```python
from build123d import *

# Parameters (mm, degrees)
EXTRUDE_1_DEPTH         = 5
SKETCH_2_R              = 14
SKETCH_2_R_2            = 12.3
EXTRUDE_2_DEPTH         = 4.5
SKETCH_3_W              = 18
SKETCH_3_H              = 18
EXTRUDE_3_DEPTH         = 3
SKETCH_4_R              = 3.6
CUT_EXTRUDE_2_DEPTH     = 24.286262044
HOLE_WIZARD_M2_1_D      = 2.4
HOLE_WIZARD_M2_1_DEPTH  = 3
HOLE_WIZARD_M2_1_TIP    = 0.721032743
CUT_EXTRUDE1_DEPTH      = 24.286262044
CUT_EXTRUDE1_DEPTH_BACK = 24.286262044
SKETCH1_R               = 1


with BuildPart() as part:
    # 스케치1 → 보스-돌출1 (new body)
    with BuildSketch(Plane.XY):
        with BuildLine():
            Line((-6, 16), (6, 16))
            ThreePointArc((6, 16), (11.656854249, 13.656854249), (14, 8))
            Line((14, 8), (14, -8))
            ThreePointArc((14, -8), (11.656854249, -13.656854249), (6, -16))
            Line((6, -16), (-6, -16))
            ThreePointArc((-6, -16), (-11.656854249, -13.656854249), (-14, -8))
            Line((-14, -8), (-14, 8))
            ThreePointArc((-14, 8), (-11.656854249, 13.656854249), (-6, 16))
        make_face()
    extrude(amount=EXTRUDE_1_DEPTH)

    # 스케치2 → 보스-돌출2 (add)
    with BuildSketch(Plane.XY.offset(5)):
        Circle(SKETCH_2_R)
        Circle(SKETCH_2_R_2, mode=Mode.SUBTRACT)
    extrude(amount=EXTRUDE_2_DEPTH)

    # 스케치3 → 보스-돌출3 (add)
    with BuildSketch(Plane(origin=(0, 0, 0), x_dir=(-1, 0, 0), z_dir=(0, 0, -1))):
        with BuildLine():
            Line((-10, 10), (-7.3, 10))
            Line((-7.3, 10), (-7.3, 14.8))
            Line((-7.3, 14.8), (-6, 14.8))
            Line((-6, 14.8), (-6, 16))
            Line((-6, 16), (6, 16))
            Line((6, 16), (6, 14.8))
            Line((6, 14.8), (7.3, 14.8))
            Line((7.3, 14.8), (7.3, 10))
            Line((7.3, 10), (10, 10))
            Line((10, 10), (10, 2.4))
            Line((10, 2.4), (11, 2.4))
            ThreePointArc((11, 2.4), (13.4, 0), (11, -2.4))
            Line((11, -2.4), (10, -2.4))
            Line((10, -2.4), (10, -10))
            Line((10, -10), (-10, -10))
            Line((-10, -10), (-10, -2.4))
            Line((-10, -2.4), (-11, -2.4))
            ThreePointArc((-11, -2.4), (-13.4, 0), (-11, 2.4))
            Line((-11, 2.4), (-10, 2.4))
            Line((-10, 2.4), (-10, 10))
        make_face()
        Rectangle(SKETCH_3_W, SKETCH_3_H, mode=Mode.SUBTRACT)
    extrude(amount=EXTRUDE_3_DEPTH)

    # 스케치4 → 컷-돌출2 (cut, through all)
    with BuildSketch(Plane.XY):
        Circle(SKETCH_4_R)
    extrude(amount=CUT_EXTRUDE_2_DEPTH, mode=Mode.SUBTRACT)

    # M2 여유 구멍1
    with Locations(Plane(origin=(-11, 0, -3), x_dir=(-1, 0, 0), z_dir=(0, 0, -1))):
        with Locations((0, 0), (-22, 0)):
            Hole(HOLE_WIZARD_M2_1_D / 2, depth=HOLE_WIZARD_M2_1_DEPTH)
            with Locations((0, 0, -(HOLE_WIZARD_M2_1_DEPTH + HOLE_WIZARD_M2_1_TIP / 2))):  # 118° drill point
                Cone(0, HOLE_WIZARD_M2_1_D / 2, HOLE_WIZARD_M2_1_TIP, mode=Mode.SUBTRACT)

    # Sketch1 → Cut-Extrude1 (cut, two sides: drawn at the far end of the back side and taken through both)
    with BuildSketch(Plane(origin=(0, 0, 0), x_dir=(1, 0, 0), z_dir=(0, 1, 0)).offset(-CUT_EXTRUDE1_DEPTH_BACK)):
        with Locations(Location((0, -7.75, 0), (0, 0, 270))):
            Circle(SKETCH1_R)
    extrude(amount=CUT_EXTRUDE1_DEPTH + CUT_EXTRUDE1_DEPTH_BACK, mode=Mode.SUBTRACT)


solid = part.part
```
Can you work these out from the model? Positions are in its coordinate system, mm. A direction names the side the tool comes from. Give positions to 0.01 mm unless a question says otherwise; leave off trailing zeros. Loops run counter-clockwise (first coordinate to the right, second up) from the corner with the lowest first, then second, coordinate; pieces in that order, holes last. Notation, with made-up numbers: M 23,80 L 33,80 A18 ccw 33,99 Z; hole C -31.5,-5 d3. An arc over 180 degrees is marked long. One line per question, with ' | ' between items. Start each with the question number.
Q1. If we section it at B-B (x = 0): State how many separate pieces and enclosed holes the cut face has, plus the area to 4 significant figures.
Q2. If we section it at A-A (z = 2.5): Please give me the cut outline in (x, y).
Q3. If we mould it in two halves opening along X, with no side actions, what happens to faces 1 (the flat face through (0, 15, 5)), 2 (the cylindrical face through (-11.594, -13.719, 2.465)), 3 (the flat face through (0, 9, -1))? For each: +X half, -X half, draft (parallel to the pull), parting line (faces both ways), or undercut.
Q4. For faces 4 (the cylindrical face through (13.4, -0.05, -1.48)), 5 (the flat face through (-6, 15, -1)), 6 (the flat face through (-10.5, -2.4, -1.5)), which set-ups out of +Z, -Z, +X, -X, +Y, -Y let a thin tool reach every point of the face, with its end or its side?
Q5. For pin 1 Ø4 at (x, y) = (-11, 0) entering from +Z; pin 2 Ø0.6 at (y, z) = (15.5, -1.5) entering from +X; pin 3 Ø1 at (x, z) = (0.5, 6.5) entering from +Y; pin 4 Ø1 at (x, z) = (-7, 5) entering from +Y, each with a flat end and sliding along its axis, tell me the tip position at first contact or that it passes through.
Q6. If I drill on line 1 (X direction, y = 0, z = -1.2); line 2 (Y direction, x = 0, z = 6); line 3 (X direction, y = 0, z = 1.95), over which ranges is the centre line in solid material (lowest first)? Write a range as from..to.
Q7. If we section it at D-D (y = 13): Please give me the cut outline in (x, z) (3 decimals).
Computed:
1) separate pieces: 4 | enclosed holes: 0 | area: 156.5 mm²
2) outline: M -14,-8 A8 ccw -6,-16 L 6,-16 A8 ccw 14,-8 L 14,8 A8 ccw 6,16 L -6,16 A8 ccw -14,8 Z; hole C 0,0 d7.2
3) face 1: draft | face 2: -X half | face 3: undercut
4) face 4: -Z, +X | face 5: -Z, -X, +Y | face 6: -Z, -X, -Y
5) pin 1: stops at z = 9.5 | pin 2: stops at x = 6 | pin 3: stops at y = 14 | pin 4: stops at y = 15.98
6) line 1: x = -13.4..-12.2, -9.8..-9, 9..9.8, 12.2..13.4 | line 2: y = -14..-12.3, 12.3..14 | line 3: x = -14..-3.6, 3.6..14
7) outline: M -12.245,0 L -7.3,0 L -7.3,-3 L 7.3,-3 L 7.3,0 L 12.245,0 L 12.245,5 L 5.196,5 L 5.196,9.5 L -5.196,9.5 L -5.196,5 L -12.245,5 Z; hole C 0,7.75 d2
